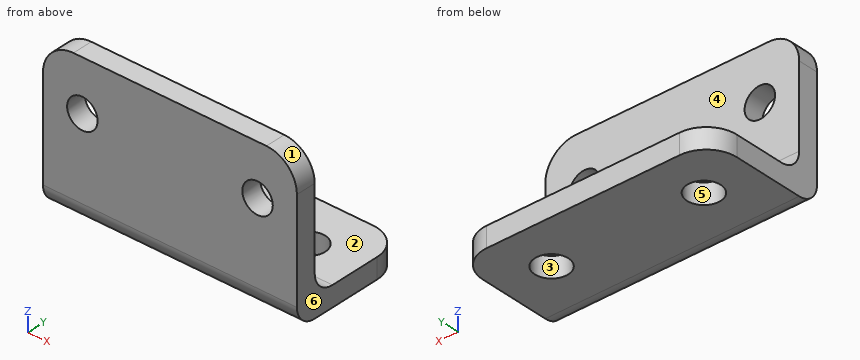
from build123d import *

# Parameters (mm, degrees)
SKETCH_R     = 1.5
PAD_DEPTH    = 2
SKETCH001_W  = 25
SKETCH001_H  = 2
PAD001_DEPTH = 10
SKETCH002_R  = 1.65
POCKET_DEPTH = 2.001
FILLET_R     = 2
FILLET001_R  = 3


with BuildPart() as part:
    # Sketch → Pad (new body)
    with BuildSketch(Plane.XZ):
        Polygon((-12.5, 5), (-12.5, -5), (-12.5, -10), (12.5, -10), (12.5, -5), (12.5, 5), align=None)
        with Locations((-8.625, 0)):
            Circle(SKETCH_R, mode=Mode.SUBTRACT)
        with Locations((8.625, 0)):
            Circle(SKETCH_R, mode=Mode.SUBTRACT)
    extrude(amount=-PAD_DEPTH)

    # Sketch001 (on Face6 of Pad) → Pad001 (join)
    with BuildSketch(Plane(origin=(0, 2, 0), x_dir=(1, 0, 0), z_dir=(0, 1, 0))):
        with Locations((0, 9)):
            Rectangle(SKETCH001_W, SKETCH001_H)
    extrude(amount=PAD001_DEPTH)

    # Sketch002 (on Face6 of Pad001) → Pocket (cut, through all)
    with BuildSketch(Plane(origin=(0, 0, -8), x_dir=(-1, 0, 0), z_dir=(0, 0, 1))):
        with Locations((-7.5, -7)):
            Circle(SKETCH002_R)
        with Locations((7.5, -7)):
            Circle(SKETCH002_R)
    extrude(amount=-POCKET_DEPTH, mode=Mode.SUBTRACT)

    # Fillet
    fillet_edges = [part.edges().sort_by_distance(p)[0] for p in [
        (0, 2, -8),
        (0, 0, -10),
    ]]
    fillet(fillet_edges, radius=FILLET_R)

    # Fillet001
    fillet001_edges = [part.edges().sort_by_distance(p)[0] for p in [
        (-12.5, 1, 5),
        (12.5, 1, 5),
        (12.5, 12, -9),
        (-12.5, 12, -9),
    ]]
    fillet(fillet001_edges, radius=FILLET001_R)


solid = part.part
Here's how the part is built. I have some questions about the finished solid (model axes, mm). Face numbers are marked on the shaded views. A direction names the side the tool comes from. Give positions to 0.01 mm unless a question says otherwise; leave off trailing zeros. Write each loop counter-clockwise with the first axis right and the second up, starting at its lowest first coordinate (ties: lowest second). Pieces come first, ordered by that corner, then holes. Notation, with made-up numbers: (65, 59) -> (71, 59) arc R23 ccw to (71, 86) -> close; hole circle Ø10 at (41.5, -34.75). An arc over 180 degrees is marked (long way). Use one line per item in the form item = value. Start each with the question number.
1. Thinking about a two-plate mould opening in Y: for the marked faces 3, 4, 5 and 6, which applies, +Y half, -Y half, draft (parallel to the pull), parting line (faces both ways), or undercut?
2. If I drill on L1, parallel to X at y = 7, z = -9.1; L2, parallel to Y at x = -4.75, z = -6; L3, parallel to Z at x = 1.75, y = 5.75, over which ranges is the centre line in solid material (lowest first)?
3. Imagine slicing it at D-D on x = 1.25. List the corners of the cut face in (y, z) for me.
4. Will these pins go through, and if not, where does the flat tip stop? pin 1 Ø2.5 at (x, z) = (-8.625, 0) entering from -Y; pin 2 Ø8 at (x, z) = (7.5, 1) entering from +Y; pin 3 Ø4.5 at (x, y) = (-7.5, 7) entering from -Z.
5. Imagine slicing it at A-A on z = 0. List the corners of the cut face in (x, y) for me (3 decimals), plus the area to 3 significant figures.
6. Imagine slicing it at C-C on x = 7.5. List the corners of the cut face in (y, z) for me, plus the area to 3 significant figures.
7. Imagine slicing it at B-B on y = 7. List the corners of the cut face in (x, z) for me, plus the area to 3 significant figures.
8. On a 3-axis mill with a long thin cutter (end or side, diameter ignored), from which of +Z, -Z, +X, -X, +Y, -Y can I reach the whole of each face in a straight line? I mean the marked faces 1 and 2. Say none if no direction works.
Entries:
q1.face_3 = undercut
q1.face_4 = +Y half
q1.face_5 = undercut
q1.face_6 = draft
q2.L1 = -12.5 to -9.15, -5.85 to 5.85, 9.15 to 12.5
q2.L2 = 0 to 2
q2.L3 = -10 to -8
q3.outline = (0, -8) arc R2 ccw to (2, -10) -> (12, -10) -> (12, -8) -> (4, -8) arc R2 cw to (2, -6) -> (2, 5) -> (0, 5) -> close
q4.pin_1 = through
q4.pin_2 = 2
q4.pin_3 = -10
q5.outline = (-12.5, 0) -> (-10.125, 0) -> (-10.125, 2) -> (-12.5, 2) -> close; (-7.125, 0) -> (7.125, 0) -> (7.125, 2) -> (-7.125, 2) -> close; (10.125, 0) -> (12.5, 0) -> (12.5, 2) -> (10.125, 2) -> close
q5.area = 38.0 mm²
q6.outline = (0, -8) arc R2 ccw to (2, -10) -> (5.35, -10) -> (5.35, -8) -> (4, -8) arc R2 cw to (2, -6) -> (2, -0.99) -> (0, -0.99) -> close; (0, 0.99) -> (2, 0.99) -> (2, 5) -> (0, 5) -> close; (8.65, -10) -> (12, -10) -> (12, -8) -> (8.65, -8) -> close
q6.area = 39.4 mm²
q7.outline = (-12.5, -10) -> (-9.15, -10) -> (-9.15, -8) -> (-12.5, -8) -> close; (-5.85, -10) -> (5.85, -10) -> (5.85, -8) -> (-5.85, -8) -> close; (9.15, -10) -> (12.5, -10) -> (12.5, -8) -> (9.15, -8) -> close
q7.area = 36.8 mm²
q8.face_1 = +Z, +X, +Y, -Y
q8.face_2 = +Z, +X, -X, +Y
